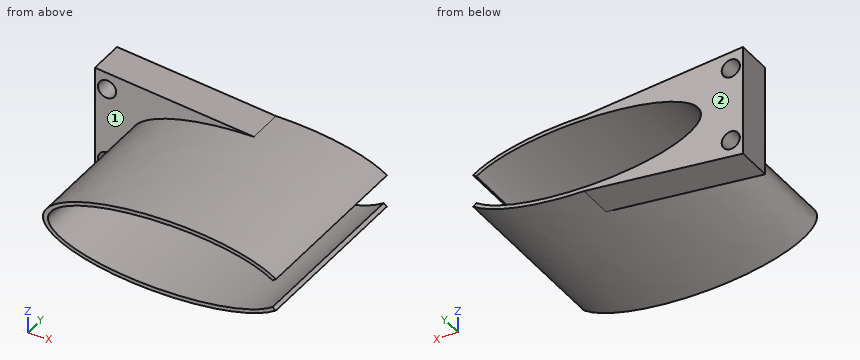
```python
from build123d import *

# Parameters (mm, degrees)
SKETCH1_RX          = 83.867123974
SKETCH1_RY          = 26.715201139
SKETCH1_RX_2        = 80.411426315
SKETCH1_RY_2        = 24.05697217
BOSS_EXTRUDE1_DEPTH = 127.254
SKETCH2_R           = 12.695879526
CUT_EXTRUDE1_DEPTH  = 157.48
BOSS_EXTRUDE2_DEPTH = 25.4
SKETCH5_R           = 6.243439839
CUT_EXTRUDE2_DEPTH  = 148.336


with BuildPart() as part:
    # Sketch1 → Boss-Extrude1 (new body)
    with BuildSketch(Plane(origin=(0, 0, 0), x_dir=(1, 0, 0), z_dir=(0, 1, 0))):
        with Locations((0, 0)):
            Ellipse(SKETCH1_RX, SKETCH1_RY)
        with Locations((0, 0)):
            Ellipse(SKETCH1_RX_2, SKETCH1_RY_2, mode=Mode.SUBTRACT)
    extrude(amount=BOSS_EXTRUDE1_DEPTH)

    # Sketch2 → Cut-Extrude1 (cut)
    with BuildSketch(Plane(origin=(0, 127.254, 0), x_dir=(1, 0, 0), z_dir=(0, 1, 0))):
        with Locations((82.362769104, 0)):
            Circle(SKETCH2_R)
    extrude(amount=-CUT_EXTRUDE1_DEPTH, mode=Mode.SUBTRACT)

    # Sketch4 → Boss-Extrude2 (add)
    with BuildSketch(Plane(origin=(0, 127.254, 0), x_dir=(1, 0, 0), z_dir=(0, 1, 0))):
        with BuildLine():
            Line((-109.288782468, 26.715201139), (-109.288782468, -26.715201139))
            Line((-109.288782468, -26.715201139), (-109.288782468, -37.805360258))
            Line((-109.288782468, -37.805360258), (0, -26.715201139))
            add(Edge.make_bspline(
                [(0, 26.715201139), (-83.867123974, 26.715201139), (-83.867123974, 0), (-83.867123974, -26.715201139), (0, -26.715201139)],
                knots=[1.570796327, 1.570796327, 1.570796327, 3.141592654, 3.141592654, 4.71238898, 4.71238898, 4.71238898], degree=2, weights=[1, 0.707106781, 1, 0.707106781, 1]))
            Line((0, 26.715201139), (-109.288782468, 38.120339295))
            Line((-109.288782468, 38.120339295), (-109.288782468, 26.715201139))
        make_face()
    extrude(amount=-BOSS_EXTRUDE2_DEPTH)

    # Sketch5 → Cut-Extrude2 (cut)
    with BuildSketch(Plane(origin=(0, 127.254, 0), x_dir=(1, 0, 0), z_dir=(0, 1, 0))):
        with Locations(Location((-100.92336604, 25.752966871, 0), (0, 0, 270))):
            Circle(SKETCH5_R)
        with Locations(Location((-100.92336604, -25.437987834, 0), (0, 0, 270))):
            Circle(SKETCH5_R)
    extrude(amount=-CUT_EXTRUDE2_DEPTH, mode=Mode.SUBTRACT)


solid = part.part
```
Here's how the part is built. I have some questions about the finished solid (model axes, mm). Face numbers are marked on the shaded views. A direction names the side the tool comes from. Coordinates: 2 decimals unless noted, no trailing zeros. Answer as CSV lines item,"result". Start each with the question number.
Q1. For the marked faces 1 and 2, which set-ups out of +Z, -Z, +X, -X, +Y, -Y let a thin tool reach every point of the face, with its end or its side?
Q2. Suppose I cut it at A-A, the plane y = 106. State how many separate pieces and enclosed holes the cut face has, then the cut area to 3 significant figures.
Q3. Will these pins go through, and if not, where does the flat tip stop? pin 1 Ø5 at (x, z) = (-39, 26.5) entering from -Y; pin 2 Ø3 at (y, z) = (13, -11) entering from -X; pin 3 Ø12 at (x, y) = (-37.5, 67) entering from -Z; pin 4 Ø11 at (x, z) = (-100.92, -25.75) entering from +Y.
Q4. I need wall thicknesses on probe 1 along Z at (x, y) = (-99, 119); probe 2 along X at (y, z) = (118.5, -14); probe 3 along Z at (x, y) = (-8, 106). Which ranges of each line are inside material? Lowest first, please. Write a range as [from, to].
Entries:
1,face 1,"-X, -Y"
1,face 2,"+Z, -Z, +X, -X, +Y"
2,separate pieces,"1"
2,enclosed holes,"2"
2,area,"4,190 mm²"
3,pin 1,"stops at y = 101.85"
3,pin 2,"stops at x = -78.39"
3,pin 3,"stops at z = -24.76"
3,pin 4,"passes through"
4,probe 1,"z = [-37.05, -31.69], [-19.81, 19.5], [31.38, 36.76]"
4,probe 2,"x = [-109.29, -65.39], [65.39, 71.43]"
4,probe 3,"z = [-27.55, -23.94], [23.94, 27.53]"
